```python
from build123d import *

# Parameters (mm, degrees)
SKETCH1_R           = 1.55
SKETCH1_R_2         = 9
SKETCH1_R_3         = 1.605
BOSS_EXTRUDE1_DEPTH = 5
SKETCH3_R           = 3.05
CUT_EXTRUDE1_DEPTH  = 2


with BuildPart() as part:
    # Sketch1 → Boss-Extrude1 (new body)
    with BuildSketch(Plane(origin=(0, 0, 0), x_dir=(1, 0, 0), z_dir=(0, 1, 0))):
        with BuildLine():
            Line((28.57509878, 48.821516158), (28.57509878, 67.821516158))
            Line((28.57509878, 67.821516158), (31.202515778, 67.821516158))
            Line((31.202515778, 67.821516158), (70.213351221, 28.810680715))
            Line((70.213351221, 28.810680715), (70.213351221, 10.832351601))
            Line((70.213351221, 10.832351601), (31.202515778, -28.178483842))
            Line((31.202515778, -28.178483842), (28.57509878, -28.178483842))
            Line((28.57509878, -28.178483842), (28.57509878, -9.178483842))
            Line((28.57509878, -9.178483842), (26.27009878, -9.178483842))
            ThreePointArc((26.27009878, -9.178483842), (25.562991999, -9.471377061), (25.27009878, -10.178483842))
            Line((25.27009878, -10.178483842), (25.27009878, -10.673483842))
            ThreePointArc((25.27009878, -10.673483842), (19.27009878, -16.673483842), (13.27009878, -10.673483842))
            Line((13.27009878, -10.673483842), (13.27009878, -10.178483842))
            ThreePointArc((13.27009878, -10.178483842), (12.977205561, -9.471377061), (12.27009878, -9.178483842))
            Line((12.27009878, -9.178483842), (-48.72490122, -9.178483842))
            Line((-48.72490122, -9.178483842), (-63.72490122, -19.178483842))
            Line((-63.72490122, -19.178483842), (-63.72490122, -9.178483842))
            Line((-63.72490122, -9.178483842), (-63.72490122, -7.077463327))
            ThreePointArc((-63.72490122, -7.077463327), (-66.610206686, -3.295840115), (-65.467541907, 1.321516158))
            ThreePointArc((-65.467541907, 1.321516158), (-66.72490122, 4.821516158), (-65.467541907, 8.321516158))
            ThreePointArc((-65.467541907, 8.321516158), (-66.72490122, 11.821516158), (-65.467541907, 15.321516158))
            ThreePointArc((-65.467541907, 15.321516158), (-66.610206686, 19.938872432), (-63.72490122, 23.720495644))
            Line((-63.72490122, 23.720495644), (-63.72490122, 48.821516158))
            Line((-63.72490122, 48.821516158), (-63.72490122, 58.821516158))
            Line((-63.72490122, 58.821516158), (-48.72490122, 48.821516158))
            Line((-48.72490122, 48.821516158), (12.27009878, 48.821516158))
            ThreePointArc((12.27009878, 48.821516158), (12.977205561, 49.114409377), (13.27009878, 49.821516158))
            Line((13.27009878, 49.821516158), (13.27009878, 50.316516158))
            ThreePointArc((13.27009878, 50.316516158), (19.27009878, 56.316516158), (25.27009878, 50.316516158))
            Line((25.27009878, 50.316516158), (25.27009878, 49.821516158))
            ThreePointArc((25.27009878, 49.821516158), (25.562991999, 49.114409377), (26.27009878, 48.821516158))
            Line((26.27009878, 48.821516158), (28.57509878, 48.821516158))
        make_face()
        with Locations(Location((26.07509878, 20.821516158, 0), (0, 0, 270))):
            Circle(SKETCH1_R, mode=Mode.SUBTRACT)
        with Locations(Location((-9.12490122, 20.821516158, 0), (0, 0, 270))):
            Circle(SKETCH1_R, mode=Mode.SUBTRACT)
        with Locations(Location((-9.12490122, 27.821516158, 0), (0, 0, 270))):
            Circle(SKETCH1_R, mode=Mode.SUBTRACT)
        with Locations(Location((26.07509878, 27.821516158, 0), (0, 0, 270))):
            Circle(SKETCH1_R, mode=Mode.SUBTRACT)
        with Locations(Location((-9.12490122, 34.821516158, 0), (0, 0, 270))):
            Circle(SKETCH1_R, mode=Mode.SUBTRACT)
        with Locations(Location((26.07509878, 34.821516158, 0), (0, 0, 270))):
            Circle(SKETCH1_R, mode=Mode.SUBTRACT)
        with Locations(Location((-9.12490122, 41.821516158, 0), (0, 0, 270))):
            Circle(SKETCH1_R, mode=Mode.SUBTRACT)
        with Locations(Location((26.07509878, 41.821516158, 0), (0, 0, 270))):
            Circle(SKETCH1_R, mode=Mode.SUBTRACT)
        with Locations(Location((-26.02490122, -2.178483842, 0), (0, 0, 270))):
            Circle(SKETCH1_R, mode=Mode.SUBTRACT)
        with Locations(Location((-61.22490122, -2.178483842, 0), (0, 0, 270))):
            Circle(SKETCH1_R, mode=Mode.SUBTRACT)
        with Locations(Location((-26.02490122, 4.821516158, 0), (0, 0, 270))):
            Circle(SKETCH1_R, mode=Mode.SUBTRACT)
        with Locations(Location((-61.22490122, 4.821516158, 0), (0, 0, 270))):
            Circle(SKETCH1_R, mode=Mode.SUBTRACT)
        with Locations(Location((-26.02490122, 11.821516158, 0), (0, 0, 270))):
            Circle(SKETCH1_R, mode=Mode.SUBTRACT)
        with Locations(Location((-61.22490122, 11.821516158, 0), (0, 0, 270))):
            Circle(SKETCH1_R, mode=Mode.SUBTRACT)
        with Locations(Location((-26.02490122, 18.821516158, 0), (0, 0, 270))):
            Circle(SKETCH1_R, mode=Mode.SUBTRACT)
        with Locations(Location((-61.22490122, 18.821516158, 0), (0, 0, 270))):
            Circle(SKETCH1_R, mode=Mode.SUBTRACT)
        with Locations(Location((-17.57490122, 39.821516158, 0), (0, 0, 270))):
            Circle(SKETCH1_R, mode=Mode.SUBTRACT)
        with Locations(Location((-17.57490122, 29.821516158, 0), (0, 0, 270))):
            Circle(SKETCH1_R, mode=Mode.SUBTRACT)
        with Locations(Location((-17.57490122, 19.821516158, 0), (0, 0, 270))):
            Circle(SKETCH1_R, mode=Mode.SUBTRACT)
        with Locations(Location((-17.57490122, 9.821516158, 0), (0, 0, 270))):
            Circle(SKETCH1_R, mode=Mode.SUBTRACT)
        with Locations(Location((-17.57490122, -0.178483842, 0), (0, 0, 270))):
            Circle(SKETCH1_R, mode=Mode.SUBTRACT)
        with Locations(Location((52.213351221, 19.821516158, 0), (0, 0, 270))):
            Circle(SKETCH1_R_2, mode=Mode.SUBTRACT)
        with Locations(Location((19.27009878, -10.673483842, 0), (0, 0, 270))):
            Circle(SKETCH1_R_3, mode=Mode.SUBTRACT)
        with Locations(Location((-44.73990122, 45.346516158, 0), (0, 0, 270))):
            Circle(SKETCH1_R_3, mode=Mode.SUBTRACT)
        with Locations(Location((38.57509878, 41.206292469, 0), (0, 0, 270))):
            Circle(SKETCH1_R, mode=Mode.SUBTRACT)
        with Locations(Location((38.57509878, -1.563260153, 0), (0, 0, 270))):
            Circle(SKETCH1_R, mode=Mode.SUBTRACT)
    extrude(amount=BOSS_EXTRUDE1_DEPTH)

    # Sketch3 → Cut-Extrude1 (cut)
    with BuildSketch(Plane(origin=(0, 0, 0), x_dir=(-1, 0, 0), z_dir=(0, -1, 0))):
        with Locations(Location((61.22490122, -2.178483842, 0), (0, 0, 90))):
            Circle(SKETCH3_R)
        with Locations(Location((61.22490122, 4.821516158, 0), (0, 0, 90))):
            Circle(SKETCH3_R)
        with Locations(Location((61.22490122, 11.821516158, 0), (0, 0, 90))):
            Circle(SKETCH3_R)
        with Locations(Location((61.22490122, 18.821516158, 0), (0, 0, 90))):
            Circle(SKETCH3_R)
        with Locations(Location((26.02490122, -2.178483842, 0), (0, 0, 90))):
            Circle(SKETCH3_R)
        with Locations(Location((26.02490122, 4.821516158, 0), (0, 0, 90))):
            Circle(SKETCH3_R)
        with Locations(Location((26.02490122, 11.821516158, 0), (0, 0, 90))):
            Circle(SKETCH3_R)
        with Locations(Location((26.02490122, 18.821516158, 0), (0, 0, 90))):
            Circle(SKETCH3_R)
        with Locations(Location((17.57490122, -0.178483842, 0), (0, 0, 90))):
            Circle(SKETCH3_R)
        with Locations(Location((17.57490122, 9.821516158, 0), (0, 0, 90))):
            Circle(SKETCH3_R)
        with Locations(Location((17.57490122, 19.821516158, 0), (0, 0, 90))):
            Circle(SKETCH3_R)
        with Locations(Location((17.57490122, 29.821516158, 0), (0, 0, 90))):
            Circle(SKETCH3_R)
        with Locations(Location((17.57490122, 39.821516158, 0), (0, 0, 90))):
            Circle(SKETCH3_R)
        with Locations(Location((9.12490122, 20.821516158, 0), (0, 0, 90))):
            Circle(SKETCH3_R)
        with Locations(Location((9.12490122, 27.821516158, 0), (0, 0, 90))):
            Circle(SKETCH3_R)
        with Locations(Location((9.12490122, 34.821516158, 0), (0, 0, 90))):
            Circle(SKETCH3_R)
        with Locations(Location((9.12490122, 41.821516158, 0), (0, 0, 90))):
            Circle(SKETCH3_R)
        with Locations(Location((-26.07509878, 20.821516158, 0), (0, 0, 90))):
            Circle(SKETCH3_R)
        with Locations(Location((-26.07509878, 27.821516158, 0), (0, 0, 90))):
            Circle(SKETCH3_R)
        with Locations(Location((-26.07509878, 34.821516158, 0), (0, 0, 90))):
            Circle(SKETCH3_R)
        with Locations(Location((-26.07509878, 41.821516158, 0), (0, 0, 90))):
            Circle(SKETCH3_R)
        with Locations(Location((-19.27009878, -10.673483842, 0), (0, 0, 90))):
            Circle(SKETCH3_R)
        with Locations(Location((44.73990122, 45.346516158, 0), (0, 0, 90))):
            Circle(SKETCH3_R)
        with Locations(Location((-38.57509878, 41.206292469, 0), (0, 0, 90))):
            Circle(SKETCH3_R)
        with Locations(Location((-38.57509878, -1.563260153, 0), (0, 0, 90))):
            Circle(SKETCH3_R)
    extrude(amount=-CUT_EXTRUDE1_DEPTH, mode=Mode.SUBTRACT)


solid = part.part
```
Geometry check sheet. Reference: the model listing, model coordinates, mm. A direction names the side the tool comes from. Give positions to 0.01 mm unless a question says otherwise; leave off trailing zeros. Order: outer loops, then holes, each group sorted by start corner. A loop starts at its lowest first (then second) coordinate and runs counter-clockwise, first axis right, second up. Notation, with made-up numbers: (49.5, -3) - (85.5, -3) arc R29 cw to (85.5, 34) - close; hole circle Ø10 at (-35.75, 31.25). An arc over 180 degrees is marked (long way). Answer in a Markdown table with one row per item. Add a question column.
Q1. Mould release check, pull along X, two halves, no side actions. Record for faces 4 (the flat face through (30, 2, -67.822)), 5 (the cylindrical face through (-66.624, 2.465, -19.871)), 6 (the flat face through (-17, 2, -28)): pulls with the +X half, pulls with the -X half, needs draft (parallel to the pull), parting line crosses it, or undercut.
Q2. Cross-section at B-B, the plane x = 1. Enter the section's corners in (y, z), then the cut area to 3 significant figures.
Q3. Cross-section at D-D, the plane x = -53. Enter the section's corners in (y, z), then the cut area to 4 significant figures.
Q4. Cross-section at A-A, the plane z = -54.5. Enter the section's corners in (x, y).
Q5. Cross-section at C-C, the plane y = 3.4. Count the separate pieces of the cut face and the enclosed holes in it, then the cut area to 3 significant figures.
Q6. Tool access check on faces 1 (the cylindrical face through (41.6, 0.99, 1.96)), 2 (the flat face through (-56.33, 2.46, -53.89)), 3 (the cylindrical face through (27.382, 3.479, -40.988)). Record the directions out of +Z, -Z, +X, -X, +Y, -Y that give a thin tool (end or side, any length) a straight path to the whole face; none if there is none.
Q7. Gauge pin test, flat ends, axial feed: pin 1 (3 mm diameter, centred on y = 1, z = -50, fed in from +X); pin 2 (3 mm diameter, centred on x = -62.5, z = -18.5, fed in from -Y); pin 3 (1.5 mm diameter, centred on x = 14, y = 1.5, fed in from +Z). Record the tip position at first contact, or that the pin passes through.
Q8. Material ranges on probe 1 along Z at (x, y) = (-44.5, 4.2); probe 2 along X at (y, z) = (2.65, -21); probe 3 along X at (y, z) = (3.45, -14), recorded low to high. Write a range as from..to.
Check values:
| question | item | result |
|---|---|---|
| 1 | face 4 | needs draft |
| 1 | face 5 | pulls with the -X half |
| 1 | face 6 | undercut |
| 2 | outline | (0, -48.82) - (5, -48.82) - (5, 9.18) - (0, 9.18) - close |
| 2 | area | 290 mm^2 |
| 3 | outline | (0, -51.67) - (5, -51.67) - (5, 12.03) - (0, 12.03) - close |
| 3 | area | 318.5 mm^2 |
| 4 | outline | (-63.72, 0) - (-57.24, 0) - (-57.24, 5) - (-63.72, 5) - close; (14.97, 0) - (23.57, 0) - (23.57, 5) - (14.97, 5) - close; (28.58, 0) - (44.52, 0) - (44.52, 5) - (28.58, 5) - close |
| 5 | separate pieces | 1 |
| 5 | enclosed holes | 26 |
| 5 | area | 7,760 mm^2 |
| 6 | face 1 | -Y |
| 6 | face 2 | -Z, +Y, -Y |
| 6 | face 3 | +Y, -Y |
| 7 | pin 1 | stops at x = 50.52 |
| 7 | pin 2 | stops at y = 2 |
| 7 | pin 3 | stops at z = 14.62 |
| 8 | probe 1 | z = -48.82..-46.93, -43.76..9.18 |
| 8 | probe 2 | x = -66.28..-18.58, -16.57..-10.66, -7.59..24.54, 27.61..43.29, 61.14..70.21 |
| 8 | probe 3 | x = -66.28..45.35, 59.08..70.21 |
